from build123d import *

# Parameters (mm, degrees)
SKETCH1_W           = 27
SKETCH1_H           = 10.8
BOSS_EXTRUDE1_DEPTH = 2
SKETCH2_W           = 27
SKETCH2_H           = 14
BOSS_EXTRUDE2_DEPTH = 2
SKETCH4_W           = 27
SKETCH4_H           = 12.8
BOSS_EXTRUDE3_DEPTH = 4
SKETCH6_W           = 11.173913912
SKETCH6_H           = 4.273360264
CUT_EXTRUDE1_DEPTH  = 24.685649664
SKETCH7_R           = 1.05
CUT_EXTRUDE2_DEPTH  = 20.519477452
SKETCH8_W           = 4.220493503
SKETCH8_H           = 6.690229829
CUT_EXTRUDE3_DEPTH  = 4
SKETCH9_W           = 4.8014854
SKETCH9_H           = 5.143985731
CUT_EXTRUDE4_DEPTH  = 4
SKETCH10_W          = 63.5
SKETCH10_H          = 31.75
BOSS_EXTRUDE5_DEPTH = 2
SKETCH11_R          = 7.036678993
SKETCH11_W          = 2.657689319
SKETCH11_H          = 6.526639736
CUT_EXTRUDE5_DEPTH  = 4
CHAMFER1_SIZE       = 10
SKETCH12_W          = 63.5
SKETCH12_H          = 1.5
BOSS_EXTRUDE6_DEPTH = 4


with BuildPart() as part:
    # Sketch1 → Boss-Extrude1 (new body)
    with BuildSketch(Plane.XY):
        Rectangle(SKETCH1_W, SKETCH1_H)
    extrude(amount=BOSS_EXTRUDE1_DEPTH)

    # Sketch2 → Boss-Extrude2 (add)
    with BuildSketch(Plane(origin=(0, 5.4, 0), x_dir=(1, 0, 0), z_dir=(0, 1, 0))):
        with Locations((0, 5)):
            Rectangle(SKETCH2_W, SKETCH2_H)
    extrude(amount=BOSS_EXTRUDE2_DEPTH)

    # Sketch4 → Boss-Extrude3 (add)
    with BuildSketch(Plane.XY.offset(2)):
        with Locations((0, 1)):
            Rectangle(SKETCH4_W, SKETCH4_H)
    extrude(amount=BOSS_EXTRUDE3_DEPTH)

    # Sketch6 → Cut-Extrude1 (cut, through all)
    with BuildSketch(Plane.XY.offset(6)):
        with Locations((7.913043044, -3.263319868)):
            Rectangle(SKETCH6_W, SKETCH6_H)
    extrude(amount=-CUT_EXTRUDE1_DEPTH, mode=Mode.SUBTRACT)

    # Sketch7 → Cut-Extrude2 (cut, through all)
    with BuildSketch(Plane(origin=(0, 0, 0), x_dir=(-1, 0, 0), z_dir=(0, 0, -1))):
        with Locations((11.7, -3.3)):
            Circle(SKETCH7_R)
        with Locations((-11.7, 3.3)):
            Circle(SKETCH7_R)
    extrude(amount=-CUT_EXTRUDE2_DEPTH, mode=Mode.SUBTRACT)

    # Sketch8 → Cut-Extrude3 (cut)
    with BuildSketch(Plane.XY.offset(6)):
        with Locations((11.389753248, 2.218475179)):
            Rectangle(SKETCH8_W, SKETCH8_H)
    extrude(amount=-CUT_EXTRUDE3_DEPTH, mode=Mode.SUBTRACT)

    # Sketch9 → Cut-Extrude4 (cut)
    with BuildSketch(Plane.XY.offset(6)):
        with Locations((-11.0992573, -2.828007134)):
            Rectangle(SKETCH9_W, SKETCH9_H)
    extrude(amount=-CUT_EXTRUDE4_DEPTH, mode=Mode.SUBTRACT)

    # Sketch10 → Boss-Extrude5 (add)
    with BuildSketch(Plane(origin=(0, 7.4, 0), x_dir=(1, 0, 0), z_dir=(0, 1, 0))):
        with Locations((0, -15.875)):
            Rectangle(SKETCH10_W, SKETCH10_H)
    extrude(amount=-BOSS_EXTRUDE5_DEPTH)

    # Sketch11 → Cut-Extrude5 (cut)
    with BuildSketch(Plane.XY.offset(2)):
        with Locations((-13.5, -5.4)):
            Circle(SKETCH11_R)
        with Locations((7.950661838, 2.136680132)):
            Rectangle(SKETCH11_W, SKETCH11_H)
    extrude(amount=CUT_EXTRUDE5_DEPTH, mode=Mode.SUBTRACT)

    # Chamfer1
    # the kernel refuses this chamfer: 10 mm, written as the material it adds along each edge
    with BuildSketch(Plane(origin=(-13.5, 5.4, 0), x_dir=(-0.9996219169112968, 0, 0.02749587661058648), z_dir=(0, 1, 0))) as chamfer1_piece_1:
        Polygon((CHAMFER1_SIZE * 0.999621916911, -CHAMFER1_SIZE * 0.0274958766106), (-CHAMFER1_SIZE * 0.0274958766106, -CHAMFER1_SIZE * 0.999621916911), (0, 0), align=None)
    extrude(amount=2)
    with BuildSketch(Plane(origin=(13.5, 7.4, 0), x_dir=(-0.027495876610586147, 0, -0.9996219169112968), z_dir=(0, -1, 0))) as chamfer1_piece_2:
        Polygon((CHAMFER1_SIZE * 0.999621916911, CHAMFER1_SIZE * 0.0274958766106), (-CHAMFER1_SIZE * 0.0274958766106, CHAMFER1_SIZE * 0.999621916911), (0, 0), align=None)
    extrude(amount=2)

    # Sketch12 → Boss-Extrude6 (add)
    with BuildSketch(Plane.XZ.offset(-5.4)):
        with Locations((0, 31)):
            Rectangle(SKETCH12_W, SKETCH12_H)
    extrude(amount=BOSS_EXTRUDE6_DEPTH)


solid = part.part
Input: part model. Units: mm. Frame: model coordinates. A direction names the side the tool comes from. Give positions to 0.01 mm unless a question says otherwise; leave off trailing zeros. Loops run counter-clockwise (first coordinate to the right, second up) from the corner with the lowest first, then second, coordinate; pieces in that order, holes last. Notation, with made-up numbers: M 66,-35 L 118,-35 A32 cw 118,4 Z; hole C 65,81 d10. An arc over 180 degrees is marked long. Use CSV: the item, a comma, the result in double quotes.
(1) Section A-A, the plane x = 11.7. Return loops of the section in (y, z).
Outcome:
outline,"M -1.13,0 L 2.25,0 L 2.25,2 L -1.13,2 Z; M 1.4,30.25 L 5.4,30.25 L 5.4,2 L 4.35,2 L 4.35,0 L 5.4,0 L 5.4,-12 L 7.4,-12 L 7.4,31.75 L 1.4,31.75 Z"
(2) Set-up query: faces 4 (the face through (-28, 6, 0)), 5 (the face through (0, 3, 30.25)), 6 (the face through (13.5, 6, -11)), 7 (the face through (10.7, 3.62, 0.99)). Return all of +Z, -Z, +X, -X, +Y, -Y with unobstructed straight access to the full face (end or side cutting, diameter ignored); none if empty.
Outcome:
face 4,"-Z, -X, +Y, -Y"
face 5,"+X, -X, -Y"
face 6,"-Z, +X, +Y, -Y"
face 7,"-Z"
(3) Material intervals for L1, parallel to Y at x = -11.7, z = 0.55; L2, parallel to Z at x = 13, y = 4.5; L3, parallel to Z at x = -2, y = -2, sorted ascending. Write a range as [from, to].
Outcome:
L1,"y = [-5.4, -4.35], [-2.25, 7.4]"
L2,"z = [0, 2], [30.25, 31.75]"
L3,"z = [0, 6]"
(4) Section C-C, the plane z = 3. Return loops of the section in (x, y), plus the area to 3 significant figures.
Outcome:
outline,"M -31.75,5.4 L -13.5,5.4 L -13.5,1.64 A7.04 cw -6.46,-5.4 L 2.33,-5.4 L 2.33,-1.13 L 6.62,-1.13 L 6.62,5.4 L 31.75,5.4 L 31.75,7.4 L -31.75,7.4 Z"
area,"287 mm²"
(5) Pin query (flat end, axial travel): P1, Ø0.6, axis at y = 6.5, z = -11, coming from the +X side; P2, Ø1.6, axis at x = 28, y = 6, coming from the -Z side; P3, Ø6.5, axis at x = 8.5, z = 2, coming from the -Y side; P4, Ø1.7, axis at x = -11.7, y = -3.3, coming from the +Z side. Return the tip coordinate at first contact, or that it passes through.
Outcome:
P1,"stops at x = 13.5"
P2,"stops at z = 0"
P3,"stops at y = -1.13"
P4,"passes through"
(6) Section B-B, the plane y = 3.3. Return loops of the section in (x, z), plus the area to 3 significant figures.
Outcome:
outline,"M -31.75,30.25 L 31.75,30.25 L 31.75,31.75 L -31.75,31.75 Z; M -13.5,0 L 10.65,0 L 10.65,2 L 6.62,2 L 6.62,6 L -13.5,6 Z; M 12.75,0 L 13.5,0 L 13.5,2 L 12.75,2 Z"
area,"226 mm²"
(7) Section D-D, the plane y = -3.3. Return loops of the section in (x, z), plus the area to 3 significant figures.
Outcome:
outline,"M -13.5,0 L -12.75,0 L -12.75,2 L -13.5,2 Z; M -10.65,0 L 2.33,0 L 2.33,6 L -6.78,6 L -6.78,2 L -10.65,2 Z"
area,"63.9 mm²"
(8) Pull-direction query (X, two-part tool) for faces 1 (the face through (-12.7, -2.98, 0.99)), 2 (the face through (0, 6, -12)), 3 (the face through (2.326, -3, 3)); classes: pulls with the +X half, pulls with the -X half, needs draft (parallel to the pull), parting line crosses it, or undercut.
Outcome:
face 1,"undercut"
face 2,"needs draft"
face 3,"pulls with the +X half"
